Part model, mm, in its own coordinate system. Round coordinates to 2 decimals unless told otherwise and drop trailing zeros. Order: outer loops, then holes, each group sorted by start corner. A loop starts at its lowest first (then second) coordinate and runs counter-clockwise, first axis right, second up. Notation, with made-up numbers: (21.5, -6.5) -> (40.5, -6.5) arc R20 ccw to (40.5, 27.5) -> close; hole circle Ø2 at (78, 34). An arc over 180 degrees is marked (long way). Use CSV: the item, a comma, the result in double quotes.
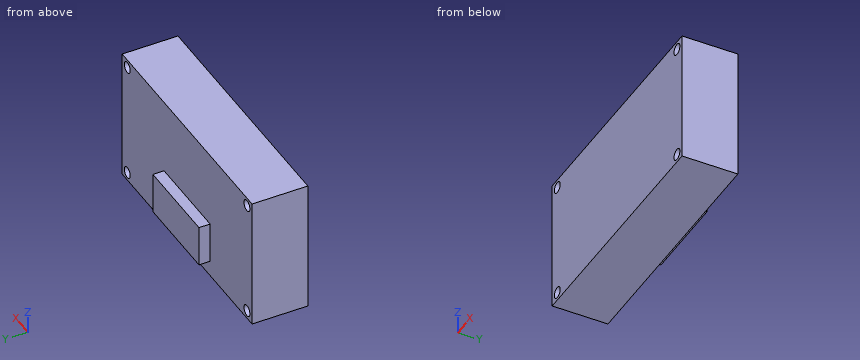
```python
from build123d import *

# Parameters (mm, degrees)
SKETCH1_W           = 66
SKETCH1_H           = 36
BOSS_EXTRUDE1_DEPTH = 15
SKETCH2_R           = 1.5
CUT_EXTRUDE1_DEPTH  = 15
SKETCH3_W           = 23.416915526
SKETCH3_H           = 11.166785339
BOSS_EXTRUDE2_DEPTH = 3


with BuildPart() as part:
    # Sketch1 → Boss-Extrude1 (new body)
    with BuildSketch(Plane(origin=(0, 0, 0), x_dir=(1, 0, 0), z_dir=(0, 1, 0))):
        Rectangle(SKETCH1_W, SKETCH1_H)
    extrude(amount=BOSS_EXTRUDE1_DEPTH)

    # Sketch2 → Cut-Extrude1 (cut)
    with BuildSketch(Plane(origin=(0, 15, 0), x_dir=(1, 0, 0), z_dir=(0, 1, 0))):
        with Locations(Location((-30.4, 15.75, 0), (0, 0, 270))):
            Circle(SKETCH2_R)
        with Locations(Location((-30.4, -15.75, 0), (0, 0, 270))):
            Circle(SKETCH2_R)
        with Locations(Location((30.4, 15.75, 0), (0, 0, 270))):
            Circle(SKETCH2_R)
        with Locations(Location((30.4, -15.75, 0), (0, 0, 270))):
            Circle(SKETCH2_R)
    extrude(amount=-CUT_EXTRUDE1_DEPTH, mode=Mode.SUBTRACT)

    # Sketch3 → Boss-Extrude2 (add)
    with BuildSketch(Plane(origin=(0, 15, 0), x_dir=(1, 0, 0), z_dir=(0, 1, 0))):
        with Locations((0, 8.102465218)):
            Rectangle(SKETCH3_W, SKETCH3_H)
    extrude(amount=BOSS_EXTRUDE2_DEPTH)


solid = part.part
```
(1) Cut at B-B, the plane z = 15.75. Give the cut face in (x, y).
Reply:
outline,"(-33, 0) -> (-31.9, 0) -> (-31.9, 15) -> (-33, 15) -> close; (-28.9, 0) -> (28.9, 0) -> (28.9, 15) -> (-28.9, 15) -> close; (31.9, 0) -> (33, 0) -> (33, 15) -> (31.9, 15) -> close"
(2) Probe probe 1 along X at (y, z) = (6.75, 15.75); probe 2 along Y at (x, z) = (17, 1). List the from-to ranges inside material, lowest first. Write a range as [from, to].
Reply:
probe 1,"[-33, -31.9], [-28.9, 28.9], [31.9, 33]"
probe 2,"[0, 15]"
(3) Cut at D-D, the plane x = 19. Give the cut face in (y, z).
Reply:
outline,"(0, -18) -> (15, -18) -> (15, 18) -> (0, 18) -> close"
(4) Cut at C-C, the plane z = -6.5. Give the cut face in (x, y).
Reply:
outline,"(-33, 0) -> (33, 0) -> (33, 15) -> (11.71, 15) -> (11.71, 18) -> (-11.71, 18) -> (-11.71, 15) -> (-33, 15) -> close"
(5) Drop flat-ended pins along their axis: P1, Ø2.5, axis at x = 0.5, y = 17, coming from the +Z side; P2, Ø12, axis at x = 14.5, z = 13.5, coming from the +Y side; P3, Ø2.5, axis at y = 16.5, z = -7.5, coming from the -X side; P4, Ø2.5, axis at x = -30.4, z = -15.75, coming from the -Y side. Give the stop position or say it passes through.
Reply:
P1,"z = -2.52"
P2,"y = 15"
P3,"x = -11.71"
P4,"through"
(6) Cut at A-A, the plane x = -30.4. Give the cut face in (y, z), then the cut area to 3 significant figures.
Reply:
outline,"(0, -18) -> (15, -18) -> (15, -17.25) -> (0, -17.25) -> close; (0, -14.25) -> (15, -14.25) -> (15, 14.25) -> (0, 14.25) -> close; (0, 17.25) -> (15, 17.25) -> (15, 18) -> (0, 18) -> close"
area,"450 mm2"
